```python
from build123d import *

# Parameters (mm, degrees)
F0_W     = 5.5195543896
F0_H     = 34.641196678
F0_R     = 2.5
F0_W_2   = 1.4996174723
F0_H_2   = 4.8834816366
F0_W_3   = 1.5
F0_H_3   = 4.1201120429
F0_H_4   = 0.1165183634
F1_DEPTH = 6


# Not quite as in the source:
# - a feature names something its author has since deleted; it is built from what else it names


with BuildPart() as f1:
    # F0 (on Top) → F1 (new body)
    with BuildSketch(Plane.XY):
        with BuildLine():
            Line((-67.1787756681, 27.2292699475), (-68.3799158582, 27.2292699475))
            ThreePointArc((-68.3799158582, 27.2292699475), (-69.0335690068, 27.1883203713), (-69.6770007567, 27.0661119853))
            ThreePointArc((-69.6770007567, 27.0661119853), (-72.5165696868, 25.2041102534), (-73.6173242331, 21.9918615726))
            Line((-73.6173242331, 21.9918615726), (-73.6173242331, -17.563536772))
            ThreePointArc((-73.6173242331, -17.563536772), (-72.0921726321, -21.2455784516), (-68.4101309525, -22.7707300525))
            Line((-68.4101309525, -22.7707300525), (61.3826757669, -22.7707300525))
            ThreePointArc((61.3826757669, -22.7707300525), (64.9182096729, -21.3062639585), (66.3826757669, -17.7707300525))
            Line((66.3826757669, -17.7707300525), (66.3826757669, 22.2292699475))
            ThreePointArc((66.3826757669, 22.2292699475), (64.9182096729, 25.7648038534), (61.3826757669, 27.2292699475))
            Line((61.3826757669, 27.2292699475), (-54.6787756681, 27.2292699475))
            Line((-54.6787756681, 27.2292699475), (-57.1787756681, 27.2292699475))
            Line((-57.1787756681, 27.2292699475), (-67.1787756681, 27.2292699475))
        make_face()
        with BuildLine():
            ThreePointArc((-68.3379918337, 19.7292699475), (-67.6057587867, 21.4970369004), (-65.8379918337, 22.2292699475))
            Line((-65.8379918337, 22.2292699475), (58.8826757669, 22.2292699475))
            ThreePointArc((58.8826757669, 22.2292699475), (60.6504427199, 21.4970369004), (61.3826757669, 19.7292699475))
            Line((61.3826757669, 19.7292699475), (61.3826757669, -15.2707300525))
            ThreePointArc((61.3826757669, -15.2707300525), (60.6504427199, -17.0384970055), (58.8826757669, -17.7707300525))
            Line((58.8826757669, -17.7707300525), (-65.8379918337, -17.7707300525))
            ThreePointArc((-65.8379918337, -17.7707300525), (-67.6057587867, -17.0384970055), (-68.3379918337, -15.2707300525))
            Line((-68.3379918337, -15.2707300525), (-68.3379918337, 19.7292699475))
        make_face(mode=Mode.SUBTRACT)
        with BuildLine():
            Line((58.8826757669, 22.2292699475), (-65.8379918337, 22.2292699475))
            ThreePointArc((-65.8379918337, 22.2292699475), (-67.6057587867, 21.4970369004), (-68.3379918337, 19.7292699475))
            Line((-68.3379918337, 19.7292699475), (-68.3379918337, -15.2707300525))
            ThreePointArc((-68.3379918337, -15.2707300525), (-67.6057587867, -17.0384970055), (-65.8379918337, -17.7707300525))
            Line((-65.8379918337, -17.7707300525), (58.8826757669, -17.7707300525))
            ThreePointArc((58.8826757669, -17.7707300525), (60.6504427199, -17.0384970055), (61.3826757669, -15.2707300525))
            Line((61.3826757669, -15.2707300525), (61.3826757669, 19.7292699475))
            ThreePointArc((61.3826757669, 19.7292699475), (60.6504427199, 21.4970369004), (58.8826757669, 22.2292699475))
        make_face()
        with BuildLine():
            ThreePointArc((-53.204651922, 0.2162606642), (-60.2757197339, 17.287328476), (-43.204651922, 10.2162606642))
            Line((-43.204651922, 10.2162606642), (-48.204651922, 10.2162606642))
            ThreePointArc((-48.204651922, 10.2162606642), (-56.7401858279, 13.7517945701), (-53.204651922, 5.2162606642))
            ThreePointArc((-53.204651922, 5.2162606642), (-46.1867208519, -11.9075475516), (-63.203530925, -4.6340106369))
            Line((-63.203530925, -4.6340106369), (-58.2024095508, -4.6340106369))
            ThreePointArc((-58.2024095508, -4.6340106369), (-49.7224574627, -8.371819846), (-53.204651922, 0.2162606642))
        make_face(mode=Mode.SUBTRACT)
        Polygon((-7.8910876493, -14.387637473), (-21.9972077757, -14.387637473), (-21.9972077757, 4.8834816366), (-21.9972077757, 5), (-18.4776540846, 5), (-16.9780366123, 5), (-7.9369102418, 5), (-7.9369102418, 4.8834816366), (-7.9369102418, -8.3816020689), (-18.8480350176, -8.3816020689), (-18.8480350176, -11.6097754424), (-7.8910876493, -11.6097754424), align=None, mode=Mode.SUBTRACT)
        Polygon((-40.7681576908, -14.7364697516), (-40.7681576908, 20.253559205), (-35.7681576908, 20.253559205), (-35.7681576908, 4.8834816366), (-25.1815660298, 4.8834816366), (-25.1776284749, 4.8834816366), (-25.1776284749, -14.387637473), (-30.1955331862, -14.387637473), (-30.1955331862, -0.1466480026), (-35.7681576908, -0.1466480026), (-35.7681576908, -14.7364697516), align=None, mode=Mode.SUBTRACT)
        Polygon((0, -14.387637473), (-4.8910876493, -14.387637473), (-4.8910876493, 4.8834816366), (0.1088994695, 4.8721321267), align=None, mode=Mode.SUBTRACT)
        Polygon((19.8960285634, -14.387637473), (11.1452508718, -14.387637473), (11.1452508718, -2.1165183634), (21.3960285634, -2.1165183634), (21.3960285634, 0.1236622645), (11.4239600822, 0.1236622645), (11.4239600822, 4.5901425229), (26.3825752896, 4.5901425229), (26.4385476336, 4.5901425229), (26.4385476336, -14.387637473), (21.3960285634, -14.387637473), align=None, mode=Mode.SUBTRACT)
        with Locations((5.7597771948, 2.932960866)):
            Rectangle(F0_W, F0_H, mode=Mode.SUBTRACT)
        with BuildLine():
            Line((47.2346405685, -14.5181566477), (42.8212322295, -14.5181566477))
            Line((42.8212322295, -14.5181566477), (42.8212322295, 4.6019549295))
            ThreePointArc((42.8212322295, 4.6019549295), (34.8761091537, 9.1588015867), (34.9547580095, 0))
            Line((34.9547580095, 0), (31.6197408739, 0))
            ThreePointArc((31.6197408739, 0), (35.1094377398, 11.6965380784), (45.0419035554, 4.6019549295))
            ThreePointArc((45.0419035554, 4.6019549295), (54.6550720871, 11.3354460366), (57.6981913518, 0))
            Line((57.6981913518, 0), (54.089111107, 0))
            ThreePointArc((54.089111107, 0), (54.9781676596, 8.7299615773), (47.2346405685, 4.6019549295))
            Line((47.2346405685, 4.6019549295), (47.2346405685, -14.5181566477))
        make_face(mode=Mode.SUBTRACT)
        with Locations((-2.6396652684, 9.5321238041)):
            Circle(F0_R, mode=Mode.SUBTRACT)
        with BuildLine():
            Line((-68.6173242331, 27.2292699475), (-68.3799158582, 27.2292699475))
            Line((-68.3799158582, 27.2292699475), (-67.1787756681, 27.2292699475))
            ThreePointArc((-67.1787756681, 27.2292699475), (-62.1787756681, 32.2292699475), (-57.1787756681, 27.2292699475))
            Line((-57.1787756681, 27.2292699475), (-54.6787756681, 27.2292699475))
            ThreePointArc((-54.6787756681, 27.2292699475), (-62.2356669727, 34.7290541697), (-69.6779125693, 27.1154906119))
            ThreePointArc((-69.6779125693, 27.1154906119), (-69.1506612176, 27.2007437391), (-68.6173242331, 27.2292699475))
        make_face()
        Polygon((-16.9780366123, 0), (-18.4776540846, 0), (-18.4776540846, -3.6654266296), (-11.7318434641, -3.6654266296), (-11.7318434641, 0), align=None)
        Polygon((14.9498761296, -10.2675254301), (19.8960285634, -10.2675254301), (21.3960285634, -10.2675254301), (21.3960285634, -7.1165183634), (14.9498761296, -7.1165183634), align=None)
        with Locations((-17.7278453484, 2.4417408183)):
            Rectangle(F0_W_2, F0_H_2)
        with Locations((20.6460285634, -12.3275814516)):
            Rectangle(F0_W_3, F0_H_3)
        with Locations((-17.7278453484, 4.9417408183)):
            Rectangle(F0_W_2, F0_H_4)
        with BuildLine():
            ThreePointArc((-69.6770007567, 27.0661119853), (-69.0335690068, 27.1883203713), (-68.3799158582, 27.2292699475))
            Line((-68.3799158582, 27.2292699475), (-68.6173242331, 27.2292699475))
            ThreePointArc((-68.6173242331, 27.2292699475), (-69.1506612176, 27.2007437391), (-69.6779125693, 27.1154906119))
            ThreePointArc((-69.6779125693, 27.1154906119), (-69.6774973076, 27.0908005481), (-69.6770007567, 27.0661119853))
        make_face()
    extrude(amount=F1_DEPTH)


solid = f1.part
```
Model file for the job. Use its own axes, mm. A direction names the side the tool comes from. Give positions to 0.01 mm unless a question says otherwise; leave off trailing zeros. Write each loop counter-clockwise with the first axis right and the second up, starting at its lowest first coordinate (ties: lowest second). Pieces come first, ordered by that corner, then holes. Notation, with made-up numbers: M -15.75,18 L 32.25,18 A11 ccw 32.25,27 Z; hole C 15.5,11.5 d10. An arc over 180 degrees is marked long. Use a Markdown table: item, result.
1) Cut at C-C (y = 2.5). Give the number of separate pieces and of enclosed holes in the cut face, and give its area (3 significant figures).
Responses:
| item | result |
|---|---|
| separate pieces | 11 |
| enclosed holes | 0 |
| area | 384 mm2 |
2) Pin check, flat tips, straight feed: pin 1 (10 mm diameter, centred on x = 49.5, y = 18.5, fed in from -Z); pin 2 (1.5 mm diameter, centred on x = -46, z = 4.5, fed in from +Y). Stop position of each tip, or through.
Responses:
| item | result |
|---|---|
| pin 1 | stops at z = 0 |
| pin 2 | stops at y = 27.23 |
3) Pull direction X, two halves, no side cores. Call faces 1 (the flat face through (-5, 6, 6)), 2 (the cylindrical face through (-72.49, 25.24, 2.96)), 3 (the flat face through (-35.768, -7, 3)), 4 (the cylindrical face through (64.879, -21.345, 2.958)): +X half, -X half, draft (parallel to the pull), parting line (faces both ways), or undercut.
Responses:
| item | result |
|---|---|
| face 1 | draft |
| face 2 | -X half |
| face 3 | undercut |
| face 4 | +X half |
4) Drill centre lines: line 1 (Y direction, x = 14, z = 3.3); line 2 (Y direction, x = -13, z = 4.8); line 3 (Y direction, x = -8, z = 1). Where is each one in solid material? Low to high. Write a range as from..to.
Responses:
| item | result |
|---|---|
| line 1 | y = -22.77..-14.39, -2.12..0.12, 4.59..27.23 |
| line 2 | y = -22.77..-14.39, -11.61..-8.38, -3.67..0, 5..27.23 |
| line 3 | y = -22.77..-14.39, -11.61..-8.38, 5..27.23 |
5) Tool access for faces 5 (the cylindrical face through (-72.132, -21.205, 2.958)), 6 (the flat face through (-62, 27.229, 3)): list every direction of +Z, -Z, +X, -X, +Y, -Y with a clear straight run to the whole face (end or side of a thin tool).
Responses:
| item | result |
|---|---|
| face 5 | +Z, -Z, -X, -Y |
| face 6 | +Z, -Z |
6) Cut at A-A (x = -28.5). List the corners of the cut face in (y, z).
Responses:
| item | result |
|---|---|
| outline | M -22.77,0 L -14.39,0 L -14.39,6 L -22.77,6 Z; M 4.88,0 L 27.23,0 L 27.23,6 L 4.88,6 Z |
7) Cut at B-B (x = -51). List the corners of the cut face in (y, z), and give its area (3 significant figures).
Responses:
| item | result |
|---|---|
| outline | M -22.77,0 L -14.54,0 L -14.54,6 L -22.77,6 Z; M -9.27,0 L -0.3,0 L -0.3,6 L -9.27,6 Z; M 4.97,0 L 14.7,0 L 14.7,6 L 4.97,6 Z; M 19.97,0 L 27.23,0 L 27.23,6 L 19.97,6 Z |
| area | 205 mm2 |
